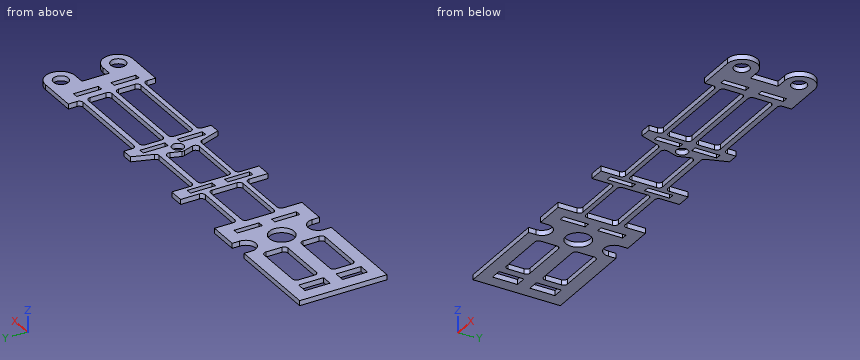
```python
from build123d import *

# Parameters (mm, degrees)
MODEL_R         = 3
MODEL_R_2       = 2.35
MODEL_R_3       = 5
MODEL_W         = 2.2
MODEL_H         = 10
MODEL_W_2       = 4.4
EXTRUDE_1_DEPTH = 2


with BuildPart() as part:
    # Model → 凸台-拉伸1 (new body)
    with BuildSketch(Plane.XY):
        with BuildLine():
            Line((42.75436257, 5.542220319), (42.75436257, 2.542220319))
            Line((42.75436257, 2.542220319), (5.024750427, 2.542220319))
            Line((5.024750427, 2.542220319), (5.024750427, 37.542220319))
            Line((5.024750427, 37.542220319), (42.75436257, 37.542220319))
            Line((42.75436257, 37.542220319), (42.75436257, 34.542220319))
            ThreePointArc((42.75436257, 34.542220319), (46.753332445, 30.45804663), (50.75230232, 34.542220319))
            Line((50.75230232, 34.542220319), (50.75230232, 37.542220319))
            Line((50.75230232, 37.542220319), (62.753332445, 37.542220319))
            Line((62.753332445, 37.542220319), (62.753332445, 30.042220319))
            ThreePointArc((62.753332445, 30.042220319), (63.192672273, 28.981560148), (64.253332445, 28.542220319))
            Line((64.253332445, 28.542220319), (84.253332445, 28.542220319))
            ThreePointArc((84.253332445, 28.542220319), (85.313992617, 28.981560148), (85.753332445, 30.042220319))
            Line((85.753332445, 30.042220319), (85.753332445, 37.542220319))
            Line((85.753332445, 37.542220319), (91.753332445, 37.542220319))
            Line((91.753332445, 37.542220319), (91.753332445, 30.042220319))
            ThreePointArc((91.753332445, 30.042220319), (92.192672273, 28.981560148), (93.253332445, 28.542220319))
            Line((93.253332445, 28.542220319), (115.596034226, 28.542220319))
            ThreePointArc((115.596034226, 28.542220319), (116.467891517, 28.821620113), (117.014953145, 29.555733833))
            Line((117.014953145, 29.555733833), (119.753177083, 37.542220319))
            Line((119.753177083, 37.542220319), (124.252549671, 37.542220319))
            Line((124.252549671, 37.542220319), (124.252549671, 34.042220319))
            ThreePointArc((124.252549671, 34.042220319), (124.6918895, 32.981560148), (125.752549671, 32.542220319))
            Line((125.752549671, 32.542220319), (160.352549671, 32.542220319))
            ThreePointArc((160.352549671, 32.542220319), (161.413209843, 32.981560148), (161.852549671, 34.042220319))
            Line((161.852549671, 34.042220319), (161.852549671, 37.542220319))
            Line((161.852549671, 37.542220319), (177.404402917, 37.542220319))
            ThreePointArc((177.404402917, 37.542220319), (183.404402917, 31.542220319), (177.404402917, 25.542220319))
            Line((177.404402917, 25.542220319), (172.92249216, 25.542220319))
            Line((172.92249216, 25.542220319), (172.92249216, 14.542220319))
            Line((172.92249216, 14.542220319), (177.404402917, 14.542220319))
            ThreePointArc((177.404402917, 14.542220319), (183.404402917, 8.542220319), (177.404402917, 2.542220319))
            Line((177.404402917, 2.542220319), (161.852549671, 2.542220319))
            Line((161.852549671, 2.542220319), (161.852549671, 6.042220319))
            ThreePointArc((161.852549671, 6.042220319), (161.413209843, 7.102880491), (160.352549671, 7.542220319))
            Line((160.352549671, 7.542220319), (125.752549671, 7.542220319))
            ThreePointArc((125.752549671, 7.542220319), (124.6918895, 7.102880491), (124.252549671, 6.042220319))
            Line((124.252549671, 6.042220319), (124.252549671, 2.542220319))
            Line((124.252549671, 2.542220319), (119.753177083, 2.542220319))
            Line((119.753177083, 2.542220319), (117.014953145, 10.528706806))
            ThreePointArc((117.014953145, 10.528706806), (116.467891517, 11.262820526), (115.596034226, 11.542220319))
            Line((115.596034226, 11.542220319), (93.253332445, 11.542220319))
            ThreePointArc((93.253332445, 11.542220319), (92.192672273, 11.102880491), (91.753332445, 10.042220319))
            Line((91.753332445, 10.042220319), (91.753332445, 2.542220319))
            Line((91.753332445, 2.542220319), (85.753332445, 2.542220319))
            Line((85.753332445, 2.542220319), (85.753332445, 10.042220319))
            ThreePointArc((85.753332445, 10.042220319), (85.313992617, 11.102880491), (84.253332445, 11.542220319))
            Line((84.253332445, 11.542220319), (64.253332445, 11.542220319))
            ThreePointArc((64.253332445, 11.542220319), (63.192672273, 11.102880491), (62.753332445, 10.042220319))
            Line((62.753332445, 10.042220319), (62.753332445, 2.542220319))
            Line((62.753332445, 2.542220319), (50.75230232, 2.542220319))
            Line((50.75230232, 2.542220319), (50.753797115, 5.474964717))
            ThreePointArc((50.753797115, 5.474964717), (46.787707643, 9.508309791), (42.75436257, 5.542220319))
        make_face()
        with Locations((177.291852583, 31.405122008)):
            Circle(MODEL_R, mode=Mode.SUBTRACT)
        with Locations((177.291852583, 8.405122008)):
            Circle(MODEL_R, mode=Mode.SUBTRACT)
        with Locations((117.403177083, 19.905122008)):
            Circle(MODEL_R_2, mode=Mode.SUBTRACT)
        with Locations((47.026395841, 19.905122008)):
            Circle(MODEL_R_3, mode=Mode.SUBTRACT)
        with Locations((57.053332445, 27.405122008)):
            Rectangle(MODEL_W, MODEL_H, mode=Mode.SUBTRACT)
        with Locations((57.053332445, 12.405122008)):
            Rectangle(MODEL_W, MODEL_H, mode=Mode.SUBTRACT)
        with Locations((165.952549671, 27.405122008)):
            Rectangle(MODEL_W, MODEL_H, mode=Mode.SUBTRACT)
        with Locations((165.952549671, 12.405122008)):
            Rectangle(MODEL_W, MODEL_H, mode=Mode.SUBTRACT)
        with Locations((120.853177083, 27.405122008)):
            Rectangle(MODEL_W, MODEL_H, mode=Mode.SUBTRACT)
        with Locations((120.853177083, 12.405122008)):
            Rectangle(MODEL_W, MODEL_H, mode=Mode.SUBTRACT)
        Polygon((87.753332445, 32.405122008), (89.953332445, 32.405122008), (89.953318849, 22.40745396), (87.753332445, 22.405122008), align=None, mode=Mode.SUBTRACT)
        Polygon((87.799905777, 7.3998381), (89.999905777, 7.3998381), (89.953262633, 17.3998381), (87.799905777, 17.3998381), align=None, mode=Mode.SUBTRACT)
        with BuildLine():
            Line((63.253332445, 26.405122008), (84.253332445, 26.405122008))
            ThreePointArc((84.253332445, 26.405122008), (85.313992617, 25.96578218), (85.753332445, 24.905122008))
            Line((85.753332445, 24.905122008), (85.753332445, 14.905122008))
            ThreePointArc((85.753332445, 14.905122008), (85.313992617, 13.844461836), (84.253332445, 13.405122008))
            Line((84.253332445, 13.405122008), (63.253332445, 13.405122008))
            ThreePointArc((63.253332445, 13.405122008), (62.192672273, 13.844461836), (61.753332445, 14.905122008))
            Line((61.753332445, 14.905122008), (61.753332445, 24.905122008))
            ThreePointArc((61.753332445, 24.905122008), (62.192672273, 25.96578218), (63.253332445, 26.405122008))
        make_face(mode=Mode.SUBTRACT)
        with BuildLine():
            Line((113.881748512, 13.405122008), (93.253332445, 13.405122008))
            ThreePointArc((93.253332445, 13.405122008), (92.192672273, 13.844461836), (91.753332445, 14.905122008))
            Line((91.753332445, 14.905122008), (91.753332445, 24.905122008))
            ThreePointArc((91.753332445, 24.905122008), (92.192672273, 25.96578218), (93.253332445, 26.405122008))
            Line((93.253332445, 26.405122008), (113.881748512, 26.405122008))
            ThreePointArc((113.881748512, 26.405122008), (115.102348719, 25.776979299), (115.300667431, 24.418635521))
            Line((115.300667431, 24.418635521), (113.91997245, 20.391608494))
            ThreePointArc((113.91997245, 20.391608494), (113.838891369, 19.905122008), (113.91997245, 19.418635521))
            Line((113.91997245, 19.418635521), (115.300667431, 15.391608494))
            ThreePointArc((115.300667431, 15.391608494), (115.102348719, 14.033264717), (113.881748512, 13.405122008))
        make_face(mode=Mode.SUBTRACT)
        with BuildLine():
            Line((161.852549671, 22.405122008), (161.852549671, 28.905122008))
            ThreePointArc((161.852549671, 28.905122008), (161.413209843, 29.96578218), (160.352549671, 30.405122008))
            Line((160.352549671, 30.405122008), (125.752549671, 30.405122008))
            ThreePointArc((125.752549671, 30.405122008), (124.6918895, 29.96578218), (124.252549671, 28.905122008))
            Line((124.252549671, 28.905122008), (124.252549671, 22.405122008))
            ThreePointArc((124.252549671, 22.405122008), (124.6918895, 21.344461836), (125.752549671, 20.905122008))
            Line((125.752549671, 20.905122008), (160.352549671, 20.905122008))
            ThreePointArc((160.352549671, 20.905122008), (161.413209843, 21.344461836), (161.852549671, 22.405122008))
        make_face(mode=Mode.SUBTRACT)
        with BuildLine():
            Line((124.252549671, 17.405122008), (124.252549671, 10.905122008))
            ThreePointArc((124.252549671, 10.905122008), (124.6918895, 9.844461836), (125.752549671, 9.405122008))
            Line((125.752549671, 9.405122008), (160.352549671, 9.405122008))
            ThreePointArc((160.352549671, 9.405122008), (161.413209843, 9.844461836), (161.852549671, 10.905122008))
            Line((161.852549671, 10.905122008), (161.852549671, 17.405122008))
            ThreePointArc((161.852549671, 17.405122008), (161.413209843, 18.46578218), (160.352549671, 18.905122008))
            Line((160.352549671, 18.905122008), (125.752549671, 18.905122008))
            ThreePointArc((125.752549671, 18.905122008), (124.6918895, 18.46578218), (124.252549671, 17.405122008))
        make_face(mode=Mode.SUBTRACT)
        with Locations((12.224750427, 27.405122008)):
            Rectangle(MODEL_W_2, MODEL_H, mode=Mode.SUBTRACT)
        with Locations((12.224750427, 12.405122008)):
            Rectangle(MODEL_W_2, MODEL_H, mode=Mode.SUBTRACT)
        with BuildLine():
            Line((19.024477888, 17.191523075), (38.228465706, 17.191523075))
            ThreePointArc((38.228465706, 17.191523075), (39.289125877, 16.752183247), (39.728465706, 15.691523075))
            Line((39.728465706, 15.691523075), (39.728465706, 9.191523075))
            ThreePointArc((39.728465706, 9.191523075), (39.289125877, 8.130862903), (38.228465706, 7.691523075))
            Line((38.228465706, 7.691523075), (19.024477888, 7.691523075))
            ThreePointArc((19.024477888, 7.691523075), (17.963817716, 8.130862903), (17.524477888, 9.191523075))
            Line((17.524477888, 9.191523075), (17.524477888, 15.691523075))
            ThreePointArc((17.524477888, 15.691523075), (17.963817716, 16.752183247), (19.024477888, 17.191523075))
        make_face(mode=Mode.SUBTRACT)
        with BuildLine():
            Line((19.024477888, 22.618720941), (38.228465706, 22.618720941))
            ThreePointArc((38.228465706, 22.618720941), (39.289125877, 23.058060769), (39.728465706, 24.118720941))
            Line((39.728465706, 24.118720941), (39.728465706, 30.618720941))
            ThreePointArc((39.728465706, 30.618720941), (39.289125877, 31.679381113), (38.228465706, 32.118720941))
            Line((38.228465706, 32.118720941), (19.024477888, 32.118720941))
            ThreePointArc((19.024477888, 32.118720941), (17.963817716, 31.679381113), (17.524477888, 30.618720941))
            Line((17.524477888, 30.618720941), (17.524477888, 24.118720941))
            ThreePointArc((17.524477888, 24.118720941), (17.963817716, 23.058060769), (19.024477888, 22.618720941))
        make_face(mode=Mode.SUBTRACT)
    extrude(amount=EXTRUDE_1_DEPTH)


solid = part.part
```
Build history of the part. All positions in model axes, mm. Give positions to 0.01 mm unless a question says otherwise; leave off trailing zeros. Loops run counter-clockwise (first coordinate to the right, second up) from the corner with the lowest first, then second, coordinate; pieces in that order, holes last.
Item 1: Drill centre lines: line 1 (Y direction, x = 30, z = 1.1); line 2 (Y direction, x = 102, z = 0.2); line 3 (Y direction, x = 128.5, z = 0.45). Where is each one in solid material? Low to high.
Answers follow:
line 1: y = 2.54 to 7.69, 17.19 to 22.62, 32.12 to 37.54
line 2: y = 11.54 to 13.41, 26.41 to 28.54
line 3: y = 7.54 to 9.41, 18.91 to 20.91, 30.41 to 32.54
Item 2: Slice it at A-A, the plane x = 66. List the corners of the cut face in (y, z), and give its area (3 significant figures).
Answers follow:
outline: (11.54, 0) - (13.41, 0) - (13.41, 2) - (11.54, 2) - close; (26.41, 0) - (28.54, 0) - (28.54, 2) - (26.41, 2) - close
area: 8.00 mm2
Item 3: Slice it at B-B, the plane x = 135. List the corners of the cut face in (y, z).
Answers follow:
outline: (7.54, 0) - (9.41, 0) - (9.41, 2) - (7.54, 2) - close; (18.91, 0) - (20.91, 0) - (20.91, 2) - (18.91, 2) - close; (30.41, 0) - (32.54, 0) - (32.54, 2) - (30.41, 2) - close
Item 4: Flat gauge pins, fed straight in: pin 1 (1 mm diameter, centred on x = 76, z = 1, fed in from +Y); pin 2 (1 mm diameter, centred on y = 11, z = 0.5, fed in from +X). Where does each tip first touch, or does it go through?
Answers follow:
pin 1: stops at y = 28.54
pin 2: stops at x = 183.08
Item 5: Slice it at C-C, the plane z = 1.65. Give the number of separate pieces and of enclosed holes in the cut face, and give its area (3 significant figures).
Answers follow:
separate pieces: 1
enclosed holes: 20
area: 2,590 mm2
